Autodesk Inventor part; units mm, degrees
ref_plane "YZ Plane" through (0, 0, 0) normal (1, 0, 0) x (0, 1, 0)
ref_plane "XZ Plane" through (0, 0, 0) normal (0, 1, 0) x (-1, 0, 0)
ref_plane "XY Plane" through (0, 0, 0) normal (0, 0, 1) x (1, 0, 0)
sketch "Sketch1" plane through (0, 0, 0) normal (0, 1, 0) x (-1, 0, 0)
  point P0 (0, 0)
sketch "Sketch2" plane through (0, 0, 0) normal (0, 0, 1) x (1, 0, 0)
  line L0 (0, 0) -> (0, 4)
  line L1 (160, 0) -> (160, 4)
  line L2 (0, 0) -> (9.95, 0)
  line L3 (160, 0) -> (150.05, 0)
  line L4 (150.05, 0) -> (150.05, 101)
  line L5 (150.05, 101) -> (9.95, 101)
  line L6 (9.95, 101) -> (9.95, 0)
  line L7 (0, 4) -> (5.95, 4)
  line L8 (5.95, 4) -> (5.95, 101)
  line L9 (5.95, 101) -> (5.95, 105)
  line L10 (5.95, 105) -> (150.05, 105)
  line L11 (150.05, 105) -> (154.05, 105)
  line L12 (154.05, 105) -> (154.05, 4)
  line L13 (154.05, 4) -> (160, 4)
  line L14 (0, 0) -> (9.95, 0)
  line L15 (150.05, 0) -> (160, 0)
extrude "Extrusion1" add sketch "Sketch2" along normal blind 250
sketch "Sketch3" plane through (5.95, 105, 0) normal (0, 1, 0) x (1, 0, 0)
  line L0 (0, 0) -> (0, -250)
  line L1 (144.1, 0) -> (144.1, -250)
  circle A0 centre (72.05, -125) radius 40
  point P0 (-5.95, 0)
  dimension "d15" = 80
extrude "Extrusion2" cut sketch "Sketch3" against normal blind 250
sketch "Sketch4" plane through (0, 0, 250) normal (0, 0, 1) x (1, 0, 0)
  point P0 (0, 0)
sketch "Sketch5" plane through (0, 0, 250) normal (0, 0, 1) x (1, 0, 0)
  line L0 (0, 0) -> (165.9252, 0)
  line L1 (165.9252, 0) -> (165.9252, 113.7831)
  line L2 (165.9252, 113.7831) -> (0, 113.7831)
  line L3 (0, 113.7831) -> (0, 0)
extrude "Extrusion3" cut sketch "Sketch5" against normal blind 50
sketch "Sketch6" plane through (0, 0, 0) normal (0, 0, -1) x (-1, 0, 0)
  line L0 (0, 4) -> (0, 0)
  line L1 (0, 0) -> (-198.2615, 0)
  line L2 (-198.2615, 0) -> (-198.2615, 123.0797)
  line L3 (-198.2615, 123.0797) -> (0, 123.0797)
  line L4 (0, 123.0797) -> (0, 0)
extrude "Extrusion4" cut sketch "Sketch6" against normal blind 40
sketch "Sketch7" plane through (160, 0, 200) normal (1, 0, 0) x (0, 0, -1)
  line L0 (0, 0) -> (0, 4)
  line L1 (160, 0) -> (0, 0)
  line L2 (0, 4) -> (160, 4)
  line L3 (160, 4) -> (160, 0)
  line L4 (160, 0) -> (0, 0)
  line L5 (0, 0) -> (0, 4)
  point P0 (200, 0)
extrude "Extrusion5" add sketch "Sketch7" along normal blind 10
sketch "Sketch8" plane through (0, 0, 200) normal (-1, 0, 0) x (0, 0, 1)
  line L0 (-160, 0) -> (0, 0)
  line L1 (-160, 4) -> (0, 4)
  line L2 (0, 4) -> (0, 0)
  line L3 (0, 0) -> (-160, 0)
  line L4 (-160, 0) -> (-160, 4)
  point P0 (-200, 0)
extrude "Extrusion6" add sketch "Sketch8" along normal blind 10
sketch "Sketch9" plane through (5.95, 4, 200) normal (0, 1, 0) x (1, 0, 0)
  line L0 (0, 160) -> (0, 0)
  line L1 (0, 0) -> (-15.95, 0)
  arc A0 (-5.475, 149.5645) -> (-10.475, 149.5645) centre (-7.975, 149.5645) ccw
  arc A1 (-10.475, 11.8823) -> (-5.475, 11.8823) centre (-7.975, 11.8823) ccw
  line L2 (-10.475, 11.8823) -> (-10.475, 149.5645)
  line L3 (-5.475, 11.8823) -> (-5.475, 149.5645)
  line L4 (164.05, 0) -> (164.05, 160)
  line L5 (164.05, 0) -> (148.5752, 0)
  line L6 (164.05, 0) -> (144.1, 0)
  line L7 (144.1, 160) -> (164.05, 160)
  arc A2 (153.8126, 11.8823) -> (158.8126, 11.8823) centre (156.3126, 11.8823) ccw
  arc A3 (158.8126, 149.5645) -> (153.8126, 149.5645) centre (156.3126, 149.5645) ccw
  line L8 (153.8126, 11.8823) -> (153.8126, 149.5645)
  line L9 (158.8126, 11.8823) -> (158.8126, 149.5645)
  point P0 (-5.95, 200)
  point P1 (-15.95, 160)
  dimension "d26" = 5
  dimension "d27" = 5
  dimension "d28" = 5
  dimension "d29" = 5
extrude "Extrusion7" cut sketch "Sketch9" against normal blind 10
sketch "Sketch10" plane through (5.95, 105, 200) normal (0, 1, 0) x (1, 0, 0)
  circle A0 centre (72.05, 75) radius 40
  line L0 (0, 0) -> (148.1, 0)
  line L1 (4, 160) -> (4, 0)
  line L2 (144.1, 160) -> (144.1, 0)
  circle A1 centre (119.55, 75) radius 5
  circle A2 centre (72.05, 27.5) radius 5
  circle A3 centre (24.55, 75) radius 5
  circle A4 centre (72.05, 122.5) radius 5
  point P0 (-5.95, 200)
  dimension "d35" = 10
  dimension "d39" = 10
  dimension "d40" = 10
  dimension "d41" = 10
extrude "Extrusion8" add sketch "Sketch10" along normal blind 10 contours A1 | A2 | A3 | A4
equation "\"BendRadius\" = Thickness"
equation "\"BendReliefWidth\" = Thickness"
equation "\"BendReliefDepth\" = 0.5 * Thickness"
equation "\"CornerReliefSize\" = 4 * Thickness"
equation "\"MinimumRemnant\" = 2 * Thickness"
equation "\"TransitionRadius\" = BendRadius"
equation "\"JacobiRadiusSize\" = BendRadius"
equation "\"GapSize\" = Thickness"
properties part number "caja"
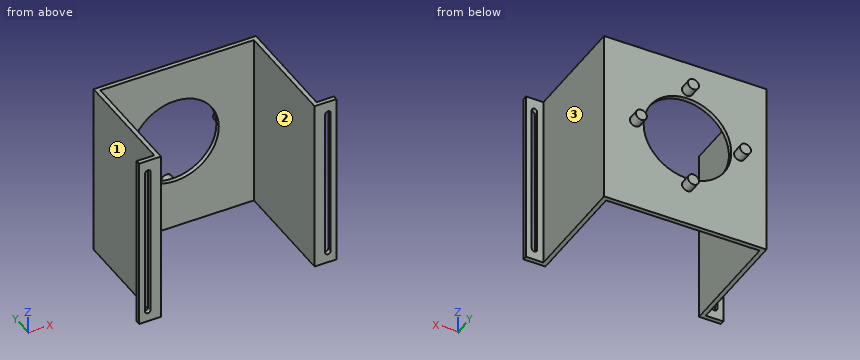
Could you check a few things on this model? Use its own coordinates, in mm. Face numbers are marked on the shaded views. Coordinates: 2 decimals unless noted, no trailing zeros. Loops run counter-clockwise (first coordinate to the right, second up) from the corner with the lowest first, then second, coordinate; pieces in that order, holes last.
1. We'd pull the mould along X, two halves only. Please class the marked faces 1, 2 and 3: released by +X, released by -X, zero draft, split by the parting line, or undercut.
2. Imagine slicing it at C-C (x = 125.5). Please give me the cut outline in (y, z).
3. Imagine slicing it at B-B (z = 60.5). Please give me the cut outline in (x, y) (3 decimals), and give its area (3 significant figures).
4. Imagine slicing it at A-A (y = 34). Please give me the cut outline in (x, z).
5. I need wall thicknesses on L1, parallel to X at y = 28.5, z = 171.5; L2, parallel to Z at x = 78, y = 103.8; L3, parallel to X at y = 103.1, z = 125. Which ranges of each line are inside material? Lowest first, please.
6. For P1, Ø5, axis at y = 19.5, z = 161.5, coming from the -X side; P2, Ø6, axis at x = 8.5, z = 88.5, coming from the +Y side; P3, Ø12, axis at y = 96.5, z = 152.5, coming from the +X side, each with a flat end and sliding along its axis, tell me the tip position at first contact or that it passes through.
7. Imagine slicing it at D-D (z = 125). Give the number of separate pieces and of enclosed holes in the cut face, and give its area (3 significant figures).
Computed values:
1. face 1: released by -X
1. face 2: undercut
1. face 3: released by +X
2. outline: (101, 40) - (105, 40) - (105, 120) - (115, 120) - (115, 130) - (105, 130) - (105, 200) - (101, 200) - close
3. outline: (-10, 0) - (-4.525, 0) - (-4.525, 4) - (-10, 4) - close; (0.475, 0) - (9.95, 0) - (9.95, 101) - (150.05, 101) - (150.05, 0) - (159.763, 0) - (159.763, 4) - (154.05, 4) - (154.05, 105) - (5.95, 105) - (5.95, 4) - (0.475, 4) - close; (164.763, 0) - (170, 0) - (170, 4) - (164.763, 4) - close
3. area: 1,490 mm2
4. outline: (5.95, 40) - (9.95, 40) - (9.95, 200) - (5.95, 200) - close; (150.05, 40) - (154.05, 40) - (154.05, 200) - (150.05, 200) - close
5. L1: x = 5.95 to 9.95, 150.05 to 154.05
5. L2: z = 40 to 85, 165 to 200
5. L3: x = 5.95 to 38, 118 to 154.05
6. P1: stops at x = 5.95
6. P2: stops at y = 105
6. P3: stops at x = 154.05
7. separate pieces: 4
7. enclosed holes: 0
7. area: 1,370 mm2
